```python
from build123d import *

# Parameters (mm, degrees)
ESBO_O1_W                = 115.09677689
ESBO_O1_H                = 52.692711406
RESSALTO_EXTRUS_O1_DEPTH = 3
ESBO_O2_R                = 1.6
CORTE_EXTRUS_O1_DEPTH    = 64.36361315
ESBO_O3_W                = 8
ESBO_O3_H                = 20
CORTE_EXTRUS_O2_DEPTH    = 64.36361315


with BuildPart() as part:
    # Esboço1 → Ressalto-extrusão1 (new body)
    with BuildSketch(Plane(origin=(0, 0, 0), x_dir=(1, 0, 0), z_dir=(0, 1, 0))):
        Rectangle(ESBO_O1_W, ESBO_O1_H)
    extrude(amount=RESSALTO_EXTRUS_O1_DEPTH)

    # Esboço2 → Corte-extrusão1 (cut, through all)
    with BuildSketch(Plane(origin=(0, 3, 0), x_dir=(1, 0, 0), z_dir=(0, 1, 0))):
        with Locations(Location((-49.548388445, 11.9, 0), (0, 0, 270))):
            Circle(ESBO_O2_R)
        with Locations(Location((-19.748388445, 11.9, 0), (0, 0, 270))):
            Circle(ESBO_O2_R)
        with Locations(Location((-49.548388445, -11.9, 0), (0, 0, 270))):
            Circle(ESBO_O2_R)
        with Locations(Location((-19.748388445, -11.9, 0), (0, 0, 270))):
            Circle(ESBO_O2_R)
        with Locations(Location((49.548388445, -11.9, 0), (0, 0, 90))):
            Circle(ESBO_O2_R)
        with Locations(Location((19.748388445, -11.9, 0), (0, 0, 90))):
            Circle(ESBO_O2_R)
        with Locations(Location((19.748388445, 11.9, 0), (0, 0, 90))):
            Circle(ESBO_O2_R)
        with Locations(Location((49.548388445, 11.9, 0), (0, 0, 90))):
            Circle(ESBO_O2_R)
    extrude(amount=-CORTE_EXTRUS_O1_DEPTH, mode=Mode.SUBTRACT)

    # Esboço3 → Corte-extrusão2 (cut, through all)
    with BuildSketch(Plane(origin=(0, 3, 0), x_dir=(1, 0, 0), z_dir=(0, 1, 0))):
        with Locations((-7.598388445, 0)):
            Rectangle(ESBO_O3_W, ESBO_O3_H)
        with Locations((7.598388445, 0)):
            Rectangle(ESBO_O3_W, ESBO_O3_H)
    extrude(amount=-CORTE_EXTRUS_O2_DEPTH, mode=Mode.SUBTRACT)


solid = part.part
```
Input: part model. Units: mm. Frame: model coordinates. A direction names the side the tool comes from. Give positions to 0.01 mm unless a question says otherwise; leave off trailing zeros. Order: outer loops, then holes, each group sorted by start corner. A loop starts at its lowest first (then second) coordinate and runs counter-clockwise, first axis right, second up. Notation, with made-up numbers: (22.5, 48) - (34.5, 48) arc R8 ccw to (34.5, 59) - close; hole circle Ø9 at (-5.5, -21). An arc over 180 degrees is marked (long way). Use a Markdown table: item, result.
(1) Draft query along X for faces 1 (the flat face through (-11.598, 2, 0)), 2 (the flat face through (57.548, 1, 0)), 3 (the flat face through (-57.548, 1, 0)). Return one class per face: released by +X, released by -X, zero draft, split by the parting line, or undercut.
Computed values:
| item | result |
|---|---|
| face 1 | undercut |
| face 2 | released by +X |
| face 3 | released by -X |
(2) Pin query (flat end, axial travel): pin 1 (3 mm diameter, centred on x = 49.55, z = -11.9, fed in from +Y). Return the tip coordinate at first contact, or that it passes through.
Computed values:
| item | result |
|---|---|
| pin 1 | passes through |
(3) Section query B-B (z = -8). Output: boundary loops of the cut face in (x, y).
Computed values:
| item | result |
|---|---|
| outline | (-57.55, 0) - (-11.6, 0) - (-11.6, 3) - (-57.55, 3) - close; (-3.6, 0) - (3.6, 0) - (3.6, 3) - (-3.6, 3) - close; (11.6, 0) - (57.55, 0) - (57.55, 3) - (11.6, 3) - close |
(4) Access query for faces 4 (the flat face through (-1, 1, -26.346)), 5 (the flat face through (8, 2, 10)). Directions: +Z, -Z, +X, -X, +Y, -Y. A direction counts if a zero-diameter tool reaches every point of the face in a straight line with its end or side. Return the directions, or none.
Computed values:
| item | result |
|---|---|
| face 4 | -Z, +X, -X, +Y, -Y |
| face 5 | +Y, -Y |
(5) Section query A-A (z = 11.9). Output: boundary loops of the cut face in (x, y).
Computed values:
| item | result |
|---|---|
| outline | (-57.55, 0) - (-51.15, 0) - (-51.15, 3) - (-57.55, 3) - close; (-47.95, 0) - (-21.35, 0) - (-21.35, 3) - (-47.95, 3) - close; (-18.15, 0) - (18.15, 0) - (18.15, 3) - (-18.15, 3) - close; (21.35, 0) - (47.95, 0) - (47.95, 3) - (21.35, 3) - close; (51.15, 0) - (57.55, 0) - (57.55, 3) - (51.15, 3) - close |
(6) Line query: line 1 (X direction, y = 2.8, z = 7); line 2 (X direction, y = 1, z = 11.9). Output: solid intervals per line, ascending. Write a range as from..to.
Computed values:
| item | result |
|---|---|
| line 1 | x = -57.55..-11.6, -3.6..3.6, 11.6..57.55 |
| line 2 | x = -57.55..-51.15, -47.95..-21.35, -18.15..18.15, 21.35..47.95, 51.15..57.55 |
(7) Section query C-C (y = 1). State how many separate pieces and enclosed holes the cut face has, then the cut area to 3 significant figures.
Computed values:
| item | result |
|---|---|
| separate pieces | 1 |
| enclosed holes | 10 |
| area | 5,680 mm2 |
